from build123d import *

# Parameters (mm, degrees)
CHAMFER5_SIZE = 0.5
SKETCH3_W     = 0.15
SKETCH3_H     = 0.8


with BuildPart() as part:
    # Sketch1 → Revolve1 (revolve)
    with BuildSketch(Plane.XY):
        Polygon((0, -16.9), (-3.175, -16.9), (-3.175, 16), (-4, 16), (-4, 26), (-5, 26), (-5, 30), (0, 30), (0, 18.825290935), align=None)
    revolve(axis=Axis((0, 55, 0), (0, -1, 0)))

    # Sketch2 → Cut-Revolve1 (revolve, cut)
    with BuildSketch(Plane.XY):
        Polygon((-3, -2.9), (-3.175, 1.1), (-3.175, -3.698889695), (-3.175, -16.9), (-3, -16.9), align=None)
    revolve(axis=Axis((0, 55, 0), (0, -1, 0)), mode=Mode.SUBTRACT)

    # Chamfer5
    chamfer5_edges = [part.edges().sort_by_distance(p)[0] for p in [
        (3, -16.9, 0),
    ]]
    chamfer(chamfer5_edges, length=CHAMFER5_SIZE)

    # Sketch3 → Cut-Revolve2 (revolve, cut)
    with BuildSketch(Plane(origin=(0, 0, 0), x_dir=(0, 0, -1), z_dir=(1, 0, 0))):
        with Locations((2.925, -15.3)):
            Rectangle(SKETCH3_W, SKETCH3_H)
    revolve(axis=Axis((0, 55, 0), (0, -1, 0)), mode=Mode.SUBTRACT)


solid = part.part
Verification items for the finished model (mm, model axes). A direction names the side the tool comes from. Round coordinates to 2 decimals unless told otherwise and drop trailing zeros. Loops run counter-clockwise (first coordinate to the right, second up) from the corner with the lowest first, then second, coordinate; pieces in that order, holes last. Notation, with made-up numbers: (-10, 5.5) - (46, 5.5) arc R25 cw to (46, 41.5) - close; hole circle Ø7 at (-23.75, -34). An arc over 180 degrees is marked (long way). Use a Markdown table: item, result. Add a question column.
1. Gauge pin test, flat ends, axial feed: pin 1 (1 mm diameter, centred on x = -3, y = 6.5, fed in from +Z); pin 2 (4 mm diameter, centred on y = -10.5, z = 1, fed in from -X); pin 3 (5 mm diameter, centred on y = -10.5, z = 2, fed in from +X). Record the tip position at first contact, or that the pin passes through.
2. Section check D-D, the plane y = 17.5. Record the boundary of the cut face in (x, z).
3. Release check for a two-part mould opening along Y. For faces 3 (the face through (1.08, 28.03, 4.88)), 4 (the face through (-1.734, -15.294, 2.262)), 5 (the face through (-3, 16, -2)), 6 (the face through (0, 30, 0)) record: released by +Y, released by -Y, zero draft, split by the parting line, or undercut.
4. Section check C-C, the plane y = -11. Record the boundary of the cut face in (x, z), plus the area to 3 significant figures.
5. Thickness scan on probe 1 along Z at (x, y) = (-4, 28); probe 2 along Y at (x, z) = (4, -2.5); probe 3 along Y at (x, z) = (-0.5, -3.25). Record the ranges inside material, lowest first. Write a range as [from, to].
6. Section check A-A, the plane x = 0. Record the boundary of the cut face in (y, z) (3 decimals), plus the area to 3 significant figures.
7. Section check B-B, the plane z = 0. Record the boundary of the cut face in (x, y) (3 decimals), plus the area to 3 significant figures.
8. Access from +Z, -Z, +X, -X, +Y, -Y to the whole of each face (thin tool, end or side, straight path). Record for faces 1 (the face through (0.867, 21.07, 3.905)), 2 (the face through (0, -16.9, 0)).
Checks:
| question | item | result |
|---|---|---|
| 1 | pin 1 | stops at z = 1.96 |
| 1 | pin 2 | stops at x = -3 |
| 1 | pin 3 | stops at x = 3 |
| 2 | outline | circle Ø8 at (0, 0) |
| 3 | face 3 | zero draft |
| 3 | face 4 | undercut |
| 3 | face 5 | released by -Y |
| 3 | face 6 | released by +Y |
| 4 | outline | circle Ø6 at (0, 0) |
| 4 | area | 28.3 mm^2 |
| 5 | probe 1 | z = [-3, 3] |
| 5 | probe 2 | y = [26, 30] |
| 5 | probe 3 | y = [16, 30] |
| 6 | outline | (-16.9, -2.5) - (-16.4, -3) - (-15.7, -3) - (-15.7, -2.85) - (-14.9, -2.85) - (-14.9, -3) - (-2.9, -3) - (1.1, -3.175) - (16, -3.175) - (16, -4) - (26, -4) - (26, -5) - (30, -5) - (30, 5) - (26, 5) - (26, 4) - (16, 4) - (16, 3.175) - (1.1, 3.175) - (-2.9, 3) - (-14.9, 3) - (-14.9, 2.85) - (-15.7, 2.85) - (-15.7, 3) - (-16.4, 3) - (-16.9, 2.5) - close |
| 6 | area | 323 mm^2 |
| 7 | outline | (-5, 26) - (-4, 26) - (-4, 16) - (-3.175, 16) - (-3.175, 1.1) - (-3, -2.9) - (-3, -14.9) - (-2.85, -14.9) - (-2.85, -15.7) - (-3, -15.7) - (-3, -16.4) - (-2.5, -16.9) - (2.5, -16.9) - (3, -16.4) - (3, -15.7) - (2.85, -15.7) - (2.85, -14.9) - (3, -14.9) - (3, -2.9) - (3.175, 1.1) - (3.175, 16) - (4, 16) - (4, 26) - (5, 26) - (5, 30) - (-5, 30) - close |
| 7 | area | 323 mm^2 |
| 8 | face 1 | -Y |
| 8 | face 2 | +Z, -Z, +X, -X, -Y |
